For this review, take the finished solid that the model builds, in its own axes (mm). Coordinates: 2 decimals unless noted, no trailing zeros. Loops run counter-clockwise (first coordinate to the right, second up) from the corner with the lowest first, then second, coordinate; pieces in that order, holes last. Notation, with made-up numbers: (3.25, 74) -> (10.25, 74) arc R22 ccw to (10.25, 94) -> close; hole circle Ø4 at (52.25, 13.25). An arc over 180 degrees is marked (long way). Answer in a Markdown table with one row per item.
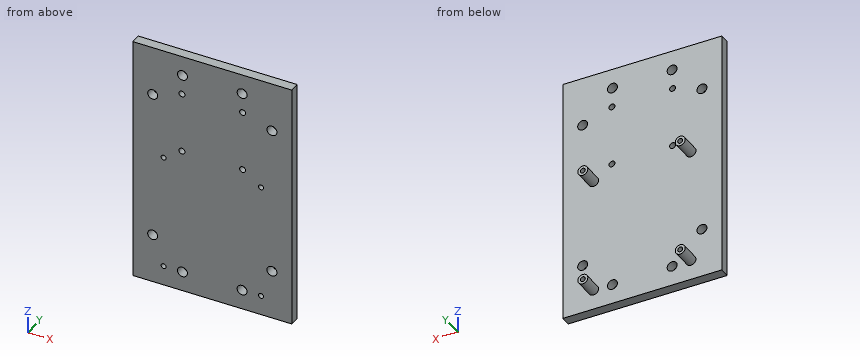
from build123d import *

# Parameters (mm, degrees)
SKETCH1_W           = 80
SKETCH1_H           = 125
SKETCH1_R           = 1.25
SKETCH1_R_2         = 1.5
BOSS_EXTRUDE1_DEPTH = 5
SKETCH2_R           = 2.5
CUT_EXTRUDE1_DEPTH  = 5
SKETCH3_R           = 2.5
SKETCH3_R_2         = 1.25
BOSS_EXTRUDE2_DEPTH = 10


with BuildPart() as part:
    # Sketch1 → Boss-Extrude1 (new body)
    with BuildSketch(Plane(origin=(0, 0, 0), x_dir=(1, 0, 0), z_dir=(0, 1, 0))):
        Rectangle(SKETCH1_W, SKETCH1_H)
        with Locations((-24.5, 52.5)):
            Circle(SKETCH1_R, mode=Mode.SUBTRACT)
        with Locations((24.5, 52.5)):
            Circle(SKETCH1_R, mode=Mode.SUBTRACT)
        with Locations((-24.5, -5.5)):
            Circle(SKETCH1_R, mode=Mode.SUBTRACT)
        with Locations((24.5, -5.5)):
            Circle(SKETCH1_R, mode=Mode.SUBTRACT)
        with Locations((-15.25, -12)):
            Circle(SKETCH1_R_2, mode=Mode.SUBTRACT)
        with Locations((15.25, -12)):
            Circle(SKETCH1_R_2, mode=Mode.SUBTRACT)
        with Locations((-15.25, -42.5)):
            Circle(SKETCH1_R_2, mode=Mode.SUBTRACT)
        with Locations((15.25, -42.5)):
            Circle(SKETCH1_R_2, mode=Mode.SUBTRACT)
    extrude(amount=BOSS_EXTRUDE1_DEPTH)

    # Sketch2 → Cut-Extrude1 (cut)
    with BuildSketch(Plane(origin=(0, 5, 0), x_dir=(1, 0, 0), z_dir=(0, 1, 0))):
        with Locations((-15, 52.5)):
            Circle(SKETCH2_R)
        with Locations((-30, 37.5)):
            Circle(SKETCH2_R)
        with Locations((15, 52.5)):
            Circle(SKETCH2_R)
        with Locations((30, 37.5)):
            Circle(SKETCH2_R)
        with Locations((30, -37.5)):
            Circle(SKETCH2_R)
        with Locations((15, -52.5)):
            Circle(SKETCH2_R)
        with Locations((-15, -52.5)):
            Circle(SKETCH2_R)
        with Locations((-30, -37.5)):
            Circle(SKETCH2_R)
    extrude(amount=-CUT_EXTRUDE1_DEPTH, mode=Mode.SUBTRACT)

    # Sketch3 → Boss-Extrude2 (add)
    with BuildSketch(Plane(origin=(0, 5, 0), x_dir=(1, 0, 0), z_dir=(0, 1, 0))):
        with Locations((-24.5, 52.5)):
            Circle(SKETCH3_R)
        with Locations((-24.5, 52.5)):
            Circle(SKETCH3_R_2, mode=Mode.SUBTRACT)
        with Locations((24.5, 52.5)):
            Circle(SKETCH3_R)
        with Locations((24.5, 52.5)):
            Circle(SKETCH3_R_2, mode=Mode.SUBTRACT)
        with Locations((-24.5, -5.5)):
            Circle(SKETCH3_R)
        with Locations((-24.5, -5.5)):
            Circle(SKETCH3_R_2, mode=Mode.SUBTRACT)
        with Locations((24.5, -5.5)):
            Circle(SKETCH3_R)
        with Locations((24.5, -5.5)):
            Circle(SKETCH3_R_2, mode=Mode.SUBTRACT)
    extrude(amount=BOSS_EXTRUDE2_DEPTH)


solid = part.part
Item 1: Insertion check: pin 1 (24 mm diameter, centred on x = -11, z = 29.5, fed in from +Y); pin 2 (4 mm diameter, centred on x = 21.5, y = 13, fed in from -Z); pin 3 (5 mm diameter, centred on y = 9, z = 7.5, fed in from -X). Each pin has a flat end and moves straight along its axis. Give the tip position at first contact, or say it passes through.
Worked answers:
| item | result |
|---|---|
| pin 1 | y = 5 |
| pin 2 | z = -54.79 |
| pin 3 | x = -27 |
Item 2: Take a section at B-B, the plane x = -24.5. State the section outline as (y, z) points, and give its area (3 significant figures).
Worked answers:
| item | result |
|---|---|
| outline | (0, -62.5) -> (5, -62.5) -> (5, -55) -> (15, -55) -> (15, -53.75) -> (0, -53.75) -> close; (0, -51.25) -> (15, -51.25) -> (15, -50) -> (5, -50) -> (5, 3) -> (15, 3) -> (15, 4.25) -> (0, 4.25) -> close; (0, 6.75) -> (15, 6.75) -> (15, 8) -> (5, 8) -> (5, 62.5) -> (0, 62.5) -> close |
| area | 650 mm² |
Item 3: Take a section at D-D, the plane z = 52.5. State the section outline as (x, y) points, and give its area (3 significant figures).
Worked answers:
| item | result |
|---|---|
| outline | (-40, 0) -> (-17.5, 0) -> (-17.5, 5) -> (-40, 5) -> close; (-12.5, 0) -> (12.5, 0) -> (12.5, 5) -> (-12.5, 5) -> close; (17.5, 0) -> (40, 0) -> (40, 5) -> (17.5, 5) -> close |
| area | 350 mm² |
Item 4: Take a section at C-C, the plane y = 11.5. State the section outline as (x, z) points.
Worked answers:
| item | result |
|---|---|
| outline | circle Ø5 at (-24.5, -52.5); circle Ø5 at (-24.5, 5.5); circle Ø5 at (24.5, -52.5); circle Ø5 at (24.5, 5.5); hole circle Ø2.5 at (-24.5, -52.5); hole circle Ø2.5 at (-24.5, 5.5); hole circle Ø2.5 at (24.5, -52.5); hole circle Ø2.5 at (24.5, 5.5) |
Item 5: Take a section at A-A, the plane z = -52.5. State the section outline as (x, y) points.
Worked answers:
| item | result |
|---|---|
| outline | (-40, 0) -> (-25.75, 0) -> (-25.75, 15) -> (-27, 15) -> (-27, 5) -> (-40, 5) -> close; (-23.25, 0) -> (-17.5, 0) -> (-17.5, 5) -> (-22, 5) -> (-22, 15) -> (-23.25, 15) -> close; (-12.5, 0) -> (12.5, 0) -> (12.5, 5) -> (-12.5, 5) -> close; (17.5, 0) -> (23.25, 0) -> (23.25, 15) -> (22, 15) -> (22, 5) -> (17.5, 5) -> close; (25.75, 0) -> (40, 0) -> (40, 5) -> (27, 5) -> (27, 15) -> (25.75, 15) -> close |
Item 6: For L1, parallel to Z at x = -15.25, y = 2.25; L2, parallel to X at y = 1.5, z = -52.5; L3, parallel to X at y = 1.5, z = -37.5, list the stretches that pass through material, from the lowest coordinate up.
Worked answers:
| item | result |
|---|---|
| L1 | -62.5 to -54.99, -50.01 to 10.5, 13.5 to 41, 44 to 50.01, 54.99 to 62.5 |
| L2 | -40 to -25.75, -23.25 to -17.5, -12.5 to 12.5, 17.5 to 23.25, 25.75 to 40 |
| L3 | -40 to -32.5, -27.5 to 27.5, 32.5 to 40 |
